The listing builds one solid part. Answer for the finished solid, in the listing's coordinates (mm). Coordinates: 2 decimals unless noted, no trailing zeros. Loops run counter-clockwise (first coordinate to the right, second up) from the corner with the lowest first, then second, coordinate; pieces in that order, holes last. Notation, with made-up numbers: M 82.5,45.5 L 137.5,45.5 A25 ccw 137.5,65.5 Z; hole C 55.5,63 d6. An arc over 180 degrees is marked long. Answer in a Markdown table with one row per item. Add a question column.
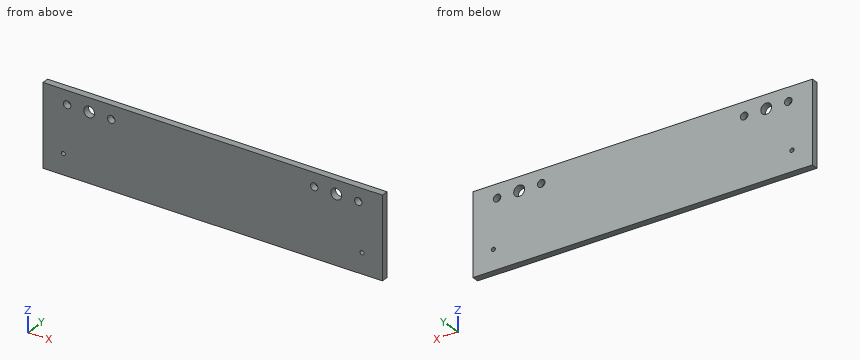
from build123d import *

# Parameters (mm, degrees)
SKETCH1_W           = 250
SKETCH1_H           = 60
SKETCH1_R           = 4
BOSS_EXTRUDE1_DEPTH = 5
SKETCH2_R           = 1.5
SKETCH2_R_2         = 2.75
CUT_EXTRUDE1_DEPTH  = 10


with BuildPart() as part:
    # Sketch1 → Boss-Extrude1 (new body)
    with BuildSketch(Plane(origin=(0, 0, 0), x_dir=(1, 0, 0), z_dir=(0, 1, 0))):
        with Locations((0, -15)):
            Rectangle(SKETCH1_W, SKETCH1_H)
        with Locations(Location((-91, -35, 0), (0, 0, 270))):
            Circle(SKETCH1_R, mode=Mode.SUBTRACT)
        with Locations(Location((91, -35, 0), (0, 0, 90))):
            Circle(SKETCH1_R, mode=Mode.SUBTRACT)
    extrude(amount=BOSS_EXTRUDE1_DEPTH)

    # Sketch2 → Cut-Extrude1 (cut)
    with BuildSketch(Plane.XZ):
        with Locations(Location((110, 0, 0), (0, 0, 270))):
            Circle(SKETCH2_R)
        with Locations(Location((74.75, 35, 0), (0, 0, 270))):
            Circle(SKETCH2_R_2)
        with Locations(Location((107.25, 35, 0), (0, 0, 270))):
            Circle(SKETCH2_R_2)
        with Locations(Location((-110, 0, 0), (0, 0, 270))):
            Circle(SKETCH2_R)
        with Locations(Location((-74.75, 35, 0), (0, 0, 270))):
            Circle(SKETCH2_R_2)
        with Locations(Location((-107.25, 35, 0), (0, 0, 270))):
            Circle(SKETCH2_R_2)
    extrude(amount=-CUT_EXTRUDE1_DEPTH, mode=Mode.SUBTRACT)


solid = part.part
(1) A cutting plane is placed at B-B (z = 35). Give the vertices of the cut face in (x, y).
(2) A cutting plane is placed at C-C (x = -91). Give the vertices of the cut face in (y, z).
(3) A cutting plane is placed at A-A (x = 74.75). Give the vertices of the cut face in (y, z), plus the area to 4 significant figures.
(4) Straight lines are drawn through the part: line 1 (X direction, y = 3.05, z = 0); line 2 (X direction, y = 3.45, z = 32). For each, find the intervals that lie inside material, in ascending order.
Solved:
| question | item | result |
|---|---|---|
| 1 | outline | M -125,0 L -110,0 L -110,5 L -125,5 Z; M -104.5,0 L -95,0 L -95,5 L -104.5,5 Z; M -87,0 L -77.5,0 L -77.5,5 L -87,5 Z; M -72,0 L 72,0 L 72,5 L -72,5 Z; M 77.5,0 L 87,0 L 87,5 L 77.5,5 Z; M 95,0 L 104.5,0 L 104.5,5 L 95,5 Z; M 110,0 L 125,0 L 125,5 L 110,5 Z |
| 2 | outline | M 0,-15 L 5,-15 L 5,31 L 0,31 Z; M 0,39 L 5,39 L 5,45 L 0,45 Z |
| 3 | outline | M 0,-15 L 5,-15 L 5,32.25 L 0,32.25 Z; M 0,37.75 L 5,37.75 L 5,45 L 0,45 Z |
| 3 | area | 272.5 mm² |
| 4 | line 1 | x = -125 to -111.5, -108.5 to 108.5, 111.5 to 125 |
| 4 | line 2 | x = -125 to -93.65, -88.35 to 88.35, 93.65 to 125 |
